Here's how the part is built. I have some questions about the finished solid (model axes, mm). Face numbers are marked on the shaded views. A direction names the side the tool comes from. Round coordinates to 2 decimals unless told otherwise and drop trailing zeros. Order: outer loops, then holes, each group sorted by start corner. A loop starts at its lowest first (then second) coordinate and runs counter-clockwise, first axis right, second up. Notation, with made-up numbers: M 72.25,-6.75 L 105.25,-6.75 A14 cw 105.25,5.25 Z; hole C -16.75,-26.5 d2. An arc over 180 degrees is marked long. Write each question's results on one line, items separated by ' | '. Start each with the question number.
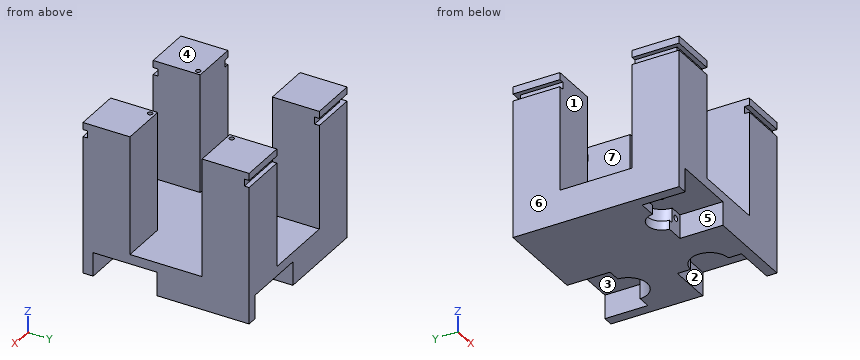
```python
from build123d import *

# Parameters (mm, degrees)
ESQUISSE1_W                  = 70
ESQUISSE1_H                  = 70
BOSS_EXTRU_1_DEPTH           = 64
ESQUISSE2_W                  = 30.4
ESQUISSE2_H                  = 19.8
ESQUISSE2_H_2                = 30.4
ESQUISSE2_W_2                = 19.8
ENL_V_MAT_EXTRU_1_DEPTH      = 50
ESQUISSE5_W                  = 3
ESQUISSE5_H                  = 2
ENL_V_MAT_EXTRU_3_DEPTH      = 71
ESQUISSE6_W                  = 2
ESQUISSE6_H                  = 3
ENL_V_MAT_EXTRU_4_DEPTH      = 71
ESQUISSE7_R                  = 1
ENL_V_MAT_EXTRU_5_DEPTH      = 65
ENL_V_MAT_EXTRU_7_DEPTH      = 10
BOSS_EXTRU_2_DEPTH           = 3.8
ESQUISSE10_W                 = 27
ESQUISSE10_H                 = 18.1
ENL_V_MAT_EXTRU_8_DEPTH      = 10
ESQUISSE11_R                 = 1.25
ENL_V_MAT_EXTRU_9_DEPTH      = 15
R_P_TITION_CIRCULAIRE1_COUNT = 3
R_P_TITION_CIRCULAIRE1_ANGLE = 180


with BuildPart() as part:
    # Esquisse1 → Boss.-Extru.1 (new body)
    with BuildSketch(Plane.XY):
        with Locations((-35, 35)):
            Rectangle(ESQUISSE1_W, ESQUISSE1_H)
    extrude(amount=BOSS_EXTRU_1_DEPTH)

    # Esquisse2 → Enlèv. mat.-Extru.1 (cut)
    with BuildSketch(Plane.XY.offset(64)):
        with Locations((-35, 60.1)):
            Rectangle(ESQUISSE2_W, ESQUISSE2_H)
        with Locations((-35, 35)):
            Rectangle(ESQUISSE2_W, ESQUISSE2_H_2)
        with Locations((-9.9, 35)):
            Rectangle(ESQUISSE2_W_2, ESQUISSE2_H_2)
        with Locations((-60.1, 35)):
            Rectangle(ESQUISSE2_W_2, ESQUISSE2_H_2)
        with Locations((-35, 9.9)):
            Rectangle(ESQUISSE2_W, ESQUISSE2_H)
    extrude(amount=-ENL_V_MAT_EXTRU_1_DEPTH, mode=Mode.SUBTRACT)

    # Esquisse5 → Enlèv. mat.-Extru.3 (cut, through all)
    with BuildSketch(Plane.ZY.offset(70)):
        with Locations((59.5, 69)):
            Rectangle(ESQUISSE5_W, ESQUISSE5_H)
        with Locations((59.5, 1)):
            Rectangle(ESQUISSE5_W, ESQUISSE5_H)
    extrude(amount=-ENL_V_MAT_EXTRU_3_DEPTH, mode=Mode.SUBTRACT)

    # Esquisse6 → Enlèv. mat.-Extru.4 (cut, through all)
    with BuildSketch(Plane(origin=(0, 70, 0), x_dir=(1, 0, 0), z_dir=(0, 1, 0))):
        with Locations((-69, -59.5)):
            Rectangle(ESQUISSE6_W, ESQUISSE6_H)
    extrude(amount=-ENL_V_MAT_EXTRU_4_DEPTH, mode=Mode.SUBTRACT)

    # Esquisse7 → Enlèv. mat.-Extru.5 (cut, through all)
    with BuildSketch(Plane.XY.offset(64)):
        with Locations((-52.2, 17.8)):
            Circle(ESQUISSE7_R)
    enl_v_mat_extru_5 = extrude(amount=-ENL_V_MAT_EXTRU_5_DEPTH, mode=Mode.SUBTRACT)

    # Esquisse8 → Enlèv. mat.-Extru.7 (cut)
    with BuildSketch(Plane(origin=(0, 0, 0), x_dir=(-1, 0, 0), z_dir=(0, 0, -1))):
        with BuildLine():
            Line((60.2, 0), (60.2, 17.8))
            ThreePointArc((60.2, 17.8), (52.2, 9.8), (44.2, 17.8))
            Line((44.2, 17.8), (44.2, 0))
            Line((44.2, 0), (60.2, 0))
        make_face()
        with BuildLine():
            ThreePointArc((44.2, 17.8), (52.2, 9.8), (60.2, 17.8))
            Line((60.2, 17.8), (53.2, 17.8))
            ThreePointArc((53.2, 17.8), (52.2, 16.8), (51.2, 17.8))
            Line((51.2, 17.8), (44.2, 17.8))
        make_face()
        with BuildLine():
            Line((53.2, 17.8), (60.2, 17.8))
            ThreePointArc((60.2, 17.8), (52.2, 25.8), (44.2, 17.8))
            Line((44.2, 17.8), (51.2, 17.8))
            ThreePointArc((51.2, 17.8), (52.2, 18.8), (53.2, 17.8))
        make_face()
    enl_v_mat_extru_7 = extrude(amount=-ENL_V_MAT_EXTRU_7_DEPTH, mode=Mode.SUBTRACT)

    # Esquisse9 → Boss.-Extru.2 (add)
    with BuildSketch(Plane(origin=(0, 0, 0), x_dir=(-1, 0, 0), z_dir=(0, 0, -1))):
        with BuildLine():
            Line((46.2, 0), (46.2, 17.8))
            ThreePointArc((46.2, 17.8), (52.2, 23.8), (58.2, 17.8))
            Line((58.2, 17.8), (58.2, 0))
            Line((58.2, 0), (60.2, 0))
            Line((60.2, 0), (60.2, 17.8))
            Line((60.2, 17.8), (60.175717696, 28.742363645))
            Line((60.175717696, 28.742363645), (44.2, 28.742363645))
            Line((44.2, 28.742363645), (44.2, 0))
            Line((44.2, 0), (46.2, 0))
        make_face()
    extrude(amount=-BOSS_EXTRU_2_DEPTH)

    # Esquisse10 → Enlèv. mat.-Extru.8 (cut)
    with BuildSketch(Plane(origin=(0, 0, 0), x_dir=(-1, 0, 0), z_dir=(0, 0, -1))):
        with Locations((52.2, 9.05)):
            Rectangle(ESQUISSE10_W, ESQUISSE10_H)
    enl_v_mat_extru_8 = extrude(amount=-ENL_V_MAT_EXTRU_8_DEPTH, mode=Mode.SUBTRACT)

    # Esquisse11 → Enlèv. mat.-Extru.9 (cut)
    with BuildSketch(Plane.XZ.offset(-18.1)):
        with Locations(Location((-41.7, 7, 0), (0, 0, 270))):  # turned: the seam where the file's is
            Circle(ESQUISSE11_R)
        with Locations(Location((-62.7, 7, 0), (0, 0, 270))):  # turned: the seam where the file's is
            Circle(ESQUISSE11_R)
    extrude(amount=-ENL_V_MAT_EXTRU_9_DEPTH, mode=Mode.SUBTRACT)

    # Répétition circulaire1: Enlèv. mat.-Extru.5, Enlèv. mat.-Extru.7, Enlèv. mat.-Extru.8 ×3 about axis
    r_p_tition_circulaire1_axis = Axis((-35, 35, 0), (0, 0, 1))
    add([enl_v_mat_extru_5.rotate(r_p_tition_circulaire1_axis, i * R_P_TITION_CIRCULAIRE1_ANGLE / (R_P_TITION_CIRCULAIRE1_COUNT - 1)) for i in range(1, R_P_TITION_CIRCULAIRE1_COUNT)], mode=Mode.SUBTRACT)
    add([enl_v_mat_extru_7.rotate(r_p_tition_circulaire1_axis, i * R_P_TITION_CIRCULAIRE1_ANGLE / (R_P_TITION_CIRCULAIRE1_COUNT - 1)) for i in range(1, R_P_TITION_CIRCULAIRE1_COUNT)], mode=Mode.SUBTRACT)
    add([enl_v_mat_extru_8.rotate(r_p_tition_circulaire1_axis, i * R_P_TITION_CIRCULAIRE1_ANGLE / (R_P_TITION_CIRCULAIRE1_COUNT - 1)) for i in range(1, R_P_TITION_CIRCULAIRE1_COUNT)], mode=Mode.SUBTRACT)


solid = part.part
```
(1) I want a section at C-C on y = 55. Write out the boundary of the cut face in (x, z).
(2) I'm going to push flat-ended pins straight in: pin 1 Ø4 at (x, y) = (-20.5, 43) entering from +Z; pin 2 Ø3 at (y, z) = (7, 4.5) entering from +X; pin 3 Ø3 at (x, z) = (-41.5, 6.5) entering from -Y. Where does each tip first touch, or does it pass through?
(3) I want a section at A-A on x = -52.2. Write out the boundary of the cut face in (y, z).
(4) If we mould it in two halves opening along X, with no side actions, what happens to the marked faces 4, 5, 6 and 7? For each: pulls with the +X half, pulls with the -X half, needs draft (parallel to the pull), parting line crosses it, or undercut.
(5) Please list where these lines run through material, in increasing order: line 1 (Y direction, x = -17.8, z = 24); line 2 (X direction, y = 52.2, z = 34.5); line 3 (X direction, y = 18, z = 48).
(6) I want a section at B-B on z = 53.5. Write out the boundary of the cut face in (x, y).
(7) On a 3-axis mill with a long thin cutter (end or side, diameter ignored), from which of +Z, -Z, +X, -X, +Y, -Y can I reach the whole of each face in a straight line? I mean the marked faces 1, 2 and 3. Say none if no direction works.
Solutions:
1) outline: M -70,0 L -31.3,0 L -31.3,10 L -4.3,10 L -4.3,0 L 0,0 L 0,64 L -19.8,64 L -19.8,14 L -50.2,14 L -50.2,64 L -70,64 L -70,61 L -68,61 L -68,58 L -70,58 Z
2) pin 1: z = 14 | pin 2: x = -18.1 | pin 3: y = 18.1
3) outline: M 0,10 L 16.8,10 L 16.8,64 L 0,64 L 0,61 L 2,61 L 2,58 L 0,58 Z; M 18.8,10 L 25.8,10 L 25.8,3.8 L 23.8,3.8 L 23.8,0 L 70,0 L 70,58 L 68,58 L 68,61 L 70,61 L 70,64 L 50.2,64 L 50.2,14 L 19.8,14 L 19.8,64 L 18.8,64 Z
4) face 4: needs draft | face 5: undercut | face 6: pulls with the -X half | face 7: undercut
5) line 1: 0 to 16.8, 18.8 to 19.8, 50.2 to 51.2, 53.2 to 70 | line 2: -70 to -50.2, -19.8 to -18.8, -16.8 to 0 | line 3: -70 to -53.18, -51.22 to -50.2, -19.8 to -18.78, -16.82 to 0
6) outline: M -70,0 L -50.2,0 L -50.2,19.8 L -70,19.8 Z; M -70,50.2 L -50.2,50.2 L -50.2,70 L -70,70 Z; M -19.8,0 L 0,0 L 0,19.8 L -19.8,19.8 Z; M -19.8,50.2 L 0,50.2 L 0,70 L -19.8,70 Z; hole C -52.2,17.8 d2; hole C -17.8,17.8 d2; hole C -17.8,52.2 d2
7) face 1: +Z, +X, -X | face 2: -Z, +X | face 3: -Z, +Y
